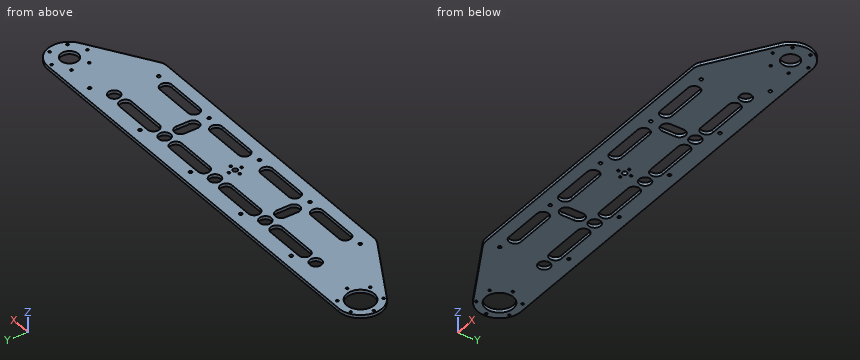
from build123d import *

# Parameters (mm, degrees)
CROQUIS2_R              = 2
CROQUIS2_R_2            = 7.5
CROQUIS2_R_3            = 17.4
CROQUIS2_R_4            = 11
CROQUIS2_R_5            = 1.5
CROQUIS2_R_6            = 3
SALIENTE_EXTRUIR1_DEPTH = 4


with BuildPart() as part:
    # Croquis2 → Saliente-Extruir1 (new body)
    with BuildSketch(Plane.XY):
        with BuildLine():
            Line((-179.195612521, -41.480204958), (179.195612521, -41.480204958))
            Line((179.195612521, -41.480204958), (190.010789857, -41.480204958))
            ThreePointArc((190.010789857, -41.480204958), (194.944809403, -40.774865591), (199.483580997, -38.715349889))
            Line((199.483580997, -38.715349889), (272.742664287, 8.031785175))
            ThreePointArc((272.742664287, 8.031785175), (286.437106864, 38.672371901), (260, 59.347542834))
            Line((260, 59.347542834), (-260, 59.347542834))
            ThreePointArc((-260, 59.347542834), (-286.437106864, 38.672371901), (-272.742664287, 8.031785175))
            Line((-272.742664287, 8.031785175), (-188.625622076, -39.240895373))
            ThreePointArc((-188.625622076, -39.240895373), (-184.06774563, -41.022236998), (-179.195612521, -41.480204958))
        make_face()
        with Locations((0, -23.892457166)):
            Circle(CROQUIS2_R, mode=Mode.SUBTRACT)
        with Locations((-90, -23.892457166)):
            Circle(CROQUIS2_R, mode=Mode.SUBTRACT)
        with Locations((-180, -23.892457166)):
            Circle(CROQUIS2_R, mode=Mode.SUBTRACT)
        with Locations((-90, 32.107542834)):
            Circle(CROQUIS2_R_2, mode=Mode.SUBTRACT)
        with Locations((0, 32.107542834)):
            Circle(CROQUIS2_R_2, mode=Mode.SUBTRACT)
        with Locations((-260, 32.107542834)):
            Circle(CROQUIS2_R_3, mode=Mode.SUBTRACT)
        with Locations(Location((260, 32.107542834, 0), (0, 0, 180))):
            Circle(CROQUIS2_R_4, mode=Mode.SUBTRACT)
        with Locations(Location((90, 32.107542834, 0), (0, 0, 180))):
            Circle(CROQUIS2_R_2, mode=Mode.SUBTRACT)
        with Locations(Location((90, -23.892457166, 0), (0, 0, 180))):
            Circle(CROQUIS2_R, mode=Mode.SUBTRACT)
        with Locations(Location((-180, 32.107542834, 0), (0, 0, 180))):
            Circle(CROQUIS2_R_2, mode=Mode.SUBTRACT)
        with Locations((180, 32.107542834)):
            Circle(CROQUIS2_R_2, mode=Mode.SUBTRACT)
        with Locations((-8, 6.607542834)):
            Circle(CROQUIS2_R_5, mode=Mode.SUBTRACT)
        with Locations((0, 14.607542834)):
            Circle(CROQUIS2_R_5, mode=Mode.SUBTRACT)
        with Locations((8, 6.607542834)):
            Circle(CROQUIS2_R_5, mode=Mode.SUBTRACT)
        with Locations((0, -1.392457166)):
            Circle(CROQUIS2_R_5, mode=Mode.SUBTRACT)
        with Locations((0, 6.607542834)):
            Circle(CROQUIS2_R_6, mode=Mode.SUBTRACT)
        with Locations((180, -23.892457166)):
            Circle(CROQUIS2_R, mode=Mode.SUBTRACT)
        with Locations((260, 9.607542834)):
            Circle(CROQUIS2_R_5, mode=Mode.SUBTRACT)
        with Locations((279.485571585, 20.857542834)):
            Circle(CROQUIS2_R_5, mode=Mode.SUBTRACT)
        with Locations((279.485571585, 43.357542834)):
            Circle(CROQUIS2_R_5, mode=Mode.SUBTRACT)
        with Locations((260, 54.607542834)):
            Circle(CROQUIS2_R_5, mode=Mode.SUBTRACT)
        with Locations((240.514428415, 43.357542834)):
            Circle(CROQUIS2_R_5, mode=Mode.SUBTRACT)
        with Locations((240.514428415, 20.857542834)):
            Circle(CROQUIS2_R_5, mode=Mode.SUBTRACT)
        with Locations((203.834428415, 46.217542834)):
            Circle(CROQUIS2_R, mode=Mode.SUBTRACT)
        with Locations((113.834428415, 46.217542834)):
            Circle(CROQUIS2_R, mode=Mode.SUBTRACT)
        with Locations((23.834428415, 46.217542834)):
            Circle(CROQUIS2_R, mode=Mode.SUBTRACT)
        with Locations((-66.165571585, 46.217542834)):
            Circle(CROQUIS2_R, mode=Mode.SUBTRACT)
        with Locations((-156.165571585, 46.217542834)):
            Circle(CROQUIS2_R, mode=Mode.SUBTRACT)
        with Locations((-248.05, 11.409535684)):
            Circle(CROQUIS2_R_5, mode=Mode.SUBTRACT)
        with Locations((-236.1, 32.107542834)):
            Circle(CROQUIS2_R_5, mode=Mode.SUBTRACT)
        with Locations((-248.05, 52.805549985)):
            Circle(CROQUIS2_R_5, mode=Mode.SUBTRACT)
        with Locations((-271.95, 52.805549985)):
            Circle(CROQUIS2_R_5, mode=Mode.SUBTRACT)
        with Locations((-283.74, 32.107542834)):
            Circle(CROQUIS2_R_5, mode=Mode.SUBTRACT)
        with Locations((-271.95, 11.409535684)):
            Circle(CROQUIS2_R_5, mode=Mode.SUBTRACT)
        with BuildLine():
            Line((-82.5, 12.107542834), (-82.5, -3.892457166))
            ThreePointArc((-82.5, -3.892457166), (-90, -11.392457166), (-97.5, -3.892457166))
            Line((-97.5, -3.892457166), (-97.5, 12.107542834))
            ThreePointArc((-97.5, 12.107542834), (-90, 19.607542834), (-82.5, 12.107542834))
        make_face(mode=Mode.SUBTRACT)
        with BuildLine():
            Line((-20, 24.607542834), (-70, 24.607542834))
            ThreePointArc((-70, 24.607542834), (-77.5, 32.107542834), (-70, 39.607542834))
            Line((-70, 39.607542834), (-20, 39.607542834))
            ThreePointArc((-20, 39.607542834), (-12.5, 32.107542834), (-20, 24.607542834))
        make_face(mode=Mode.SUBTRACT)
        with BuildLine():
            Line((160, -26.392457166), (110, -26.392457166))
            ThreePointArc((110, -26.392457166), (102.5, -18.892457166), (110, -11.392457166))
            Line((110, -11.392457166), (160, -11.392457166))
            ThreePointArc((160, -11.392457166), (167.5, -18.892457166), (160, -26.392457166))
        make_face(mode=Mode.SUBTRACT)
        with BuildLine():
            Line((20, -11.392457166), (70, -11.392457166))
            ThreePointArc((70, -11.392457166), (77.5, -18.892457166), (70, -26.392457166))
            Line((70, -26.392457166), (20, -26.392457166))
            ThreePointArc((20, -26.392457166), (12.5, -18.892457166), (20, -11.392457166))
        make_face(mode=Mode.SUBTRACT)
        with BuildLine():
            Line((20, 39.607542834), (70, 39.607542834))
            ThreePointArc((70, 39.607542834), (77.5, 32.107542834), (70, 24.607542834))
            Line((70, 24.607542834), (20, 24.607542834))
            ThreePointArc((20, 24.607542834), (12.5, 32.107542834), (20, 39.607542834))
        make_face(mode=Mode.SUBTRACT)
        with BuildLine():
            Line((-160, 39.607542834), (-110, 39.607542834))
            ThreePointArc((-110, 39.607542834), (-102.5, 32.107542834), (-110, 24.607542834))
            Line((-110, 24.607542834), (-160, 24.607542834))
            ThreePointArc((-160, 24.607542834), (-167.5, 32.107542834), (-160, 39.607542834))
        make_face(mode=Mode.SUBTRACT)
        with BuildLine():
            Line((-20, -26.392457166), (-70, -26.392457166))
            ThreePointArc((-70, -26.392457166), (-77.5, -18.892457166), (-70, -11.392457166))
            Line((-70, -11.392457166), (-20, -11.392457166))
            ThreePointArc((-20, -11.392457166), (-12.5, -18.892457166), (-20, -26.392457166))
        make_face(mode=Mode.SUBTRACT)
        with BuildLine():
            Line((160, 24.607542834), (110, 24.607542834))
            ThreePointArc((110, 24.607542834), (102.5, 32.107542834), (110, 39.607542834))
            Line((110, 39.607542834), (160, 39.607542834))
            ThreePointArc((160, 39.607542834), (167.5, 32.107542834), (160, 24.607542834))
        make_face(mode=Mode.SUBTRACT)
        with BuildLine():
            Line((-160, -26.392457166), (-110, -26.392457166))
            ThreePointArc((-110, -26.392457166), (-102.5, -18.892457166), (-110, -11.392457166))
            Line((-110, -11.392457166), (-160, -11.392457166))
            ThreePointArc((-160, -11.392457166), (-167.5, -18.892457166), (-160, -26.392457166))
        make_face(mode=Mode.SUBTRACT)
        with BuildLine():
            Line((97.5, 12.107542834), (97.5, -3.892457166))
            ThreePointArc((97.5, -3.892457166), (90, -11.392457166), (82.5, -3.892457166))
            Line((82.5, -3.892457166), (82.5, 12.107542834))
            ThreePointArc((82.5, 12.107542834), (90, 19.607542834), (97.5, 12.107542834))
        make_face(mode=Mode.SUBTRACT)
    extrude(amount=SALIENTE_EXTRUIR1_DEPTH)


solid = part.part
Read the model definition and answer for the solid it produces. Units are mm, in the model's axes. Give positions to 0.01 mm unless a question says otherwise; leave off trailing zeros. Write each loop counter-clockwise with the first axis right and the second up, starting at its lowest first coordinate (ties: lowest second). Pieces come first, ordered by that corner, then holes. Notation, with made-up numbers: (-37.75, 47) -> (-18.75, 47) arc R16 cw to (-18.75, 63) -> close; hole circle Ø6 at (13, 20.25). An arc over 180 degrees is marked (long way). Answer as a JSON object with one key per item and string values. Group by question number.
1) Consider L1, parallel to Y at x = 90, z = 3; L2, parallel to Y at x = -179.5, z = 2.8; L3, parallel to Y at x = 130.5, z = 0.55. Determine where each line is inside the solid, lowest interval first. Write a range as from..to.
2) Find section A-A (x = 233.5). Write down the section's boundary in (y, z), and give its area (3 significant figures).
3) Each of these flat-tipped pins is pushed along its axis until it touches: P1, Ø4, axis at x = 0, y = -1.39, coming from the -Z side; P2, Ø1, axis at x = -77, z = 2.5, coming from the -Y side; P3, Ø1.5, axis at y = 33, z = 3, coming from the +X side; P4, Ø3, axis at x = -180, y = -23.89, coming from the +Z side. Where does it stop, or does it pass through?
4) Find section B-B (z = 1.1). Count the separate pieces of the cut face and the enclosed holes in it, and give its area (3 significant figures).
Values follow:
{
 "1": {"L1": "y = -41.48..-25.89, -21.89..-11.39, 19.61..24.61, 39.61..59.35", "L2": "y = -41.49..-25.83, -21.96..24.62, 39.59..59.35", "L3": "y = -41.48..-26.39, -11.39..24.61, 39.61..59.35"},
 "2": {"outline": "(-17.01, 0) -> (59.35, 0) -> (59.35, 4) -> (-17.01, 4) -> close", "area": "305 mm2"},
 "3": {"P1": "stops at z = 0", "P2": "stops at y = -41.48", "P3": "stops at x = 287.24", "P4": "passes through"},
 "4": {"separate pieces": "1", "enclosed holes": "44", "area": "41,100 mm2"}
}
